Check sheet for the modelled part. Datum: model origin and axes. Units: mm. Give positions to 0.01 mm unless a question says otherwise; leave off trailing zeros. Order: outer loops, then holes, each group sorted by start corner. A loop starts at its lowest first (then second) coordinate and runs counter-clockwise, first axis right, second up. Notation, with made-up numbers: (-36, 8.25) -> (19, 8.25) arc R21 cw to (19, 22.25) -> close; hole circle Ø5 at (42.25, 45). An arc over 180 degrees is marked (long way). One line per question, with ' | ' between items.
```python
from build123d import *

# Parameters (mm, degrees)
SKETCH_1_R            = 1
SKETCH_1_R_2          = 11.2
SKETCH_1_R_3          = 4.05
SKETCH_1_R_4          = 3.5
SKETCH_1_R_5          = 8.2
SKETCH_1_R_6          = 4.2
EXTRUDE_1_DEPTH       = 7
SKETCH_6_R            = 21.8
SKETCH_6_R_2          = 8
CUT_EXTRUDE_3_DEPTH   = 4
SKETCH_7_R            = 3
CUT_EXTRUDE_4_DEPTH   = 6
SKETCH_13_R           = 1.75
CUT_EXTRUDE_4_2_DEPTH = 5


with BuildPart() as part:
    # Эскиз1 → Бобышка-Вытянуть1 (new body)
    with BuildSketch(Plane.XY):
        with BuildLine():
            Line((10, 0), (435, 0))
            ThreePointArc((435, 0), (442.071067812, 2.928932188), (445, 10))
            Line((445, 10), (445, 122.5))
            ThreePointArc((445, 122.5), (442.071067812, 129.571067812), (435, 132.5))
            Line((435, 132.5), (10, 132.5))
            ThreePointArc((10, 132.5), (2.928932188, 129.571067812), (0, 122.5))
            Line((0, 122.5), (0, 10))
            ThreePointArc((0, 10), (2.928932188, 2.928932188), (10, 0))
        make_face()
        with Locations((222.3, 105)):
            Circle(SKETCH_1_R, mode=Mode.SUBTRACT)
        with Locations((222.3, 66)):
            Circle(SKETCH_1_R_2, mode=Mode.SUBTRACT)
        with Locations((80, 66)):
            Circle(SKETCH_1_R_3, mode=Mode.SUBTRACT)
        with Locations((264, 66)):
            Circle(SKETCH_1_R_4, mode=Mode.SUBTRACT)
        with Locations((294, 66)):
            Circle(SKETCH_1_R_4, mode=Mode.SUBTRACT)
        with Locations((180.6, 66)):
            Circle(SKETCH_1_R_5, mode=Mode.SUBTRACT)
        with Locations((365, 66)):
            Circle(SKETCH_1_R_6, mode=Mode.SUBTRACT)
        with Locations((15.6, 66)):
            Circle(SKETCH_1_R_5, mode=Mode.SUBTRACT)
        with Locations((150.6, 66)):
            Circle(SKETCH_1_R_5, mode=Mode.SUBTRACT)
    extrude(amount=EXTRUDE_1_DEPTH)

    # Эскиз6 → Вырез-Вытянуть3 (cut)
    with BuildSketch(Plane.XY.offset(7)):
        with Locations((80, 66)):
            Circle(SKETCH_6_R)
        with Locations((365, 66)):
            Circle(SKETCH_6_R)
        with Locations((264, 66)):
            Circle(SKETCH_6_R_2)
        with Locations((294, 66)):
            Circle(SKETCH_6_R_2)
    extrude(amount=-CUT_EXTRUDE_3_DEPTH, mode=Mode.SUBTRACT)

    # Эскиз7 → Cut-Extrude 4 (cut)
    with BuildSketch(Plane(origin=(0, 0, 0), x_dir=(-1, 0, 0), z_dir=(0, 0, -1))):
        with Locations((-222.3, 105)):
            Circle(SKETCH_7_R)
    extrude(amount=-CUT_EXTRUDE_4_DEPTH, mode=Mode.SUBTRACT)

    # Эскиз13 → Cut-Extrude 4 2 (cut)
    with BuildSketch(Plane(origin=(0, 0, 0), x_dir=(-1, 0, 0), z_dir=(0, 0, -1))):
        with Locations((-17, 118.4)):
            Circle(SKETCH_13_R)
        with Locations((-17, 14.1)):
            Circle(SKETCH_13_R)
        with Locations((-428, 14.1)):
            Circle(SKETCH_13_R)
        with Locations((-428, 118.4)):
            Circle(SKETCH_13_R)
    extrude(amount=-CUT_EXTRUDE_4_2_DEPTH, mode=Mode.SUBTRACT)


solid = part.part
```
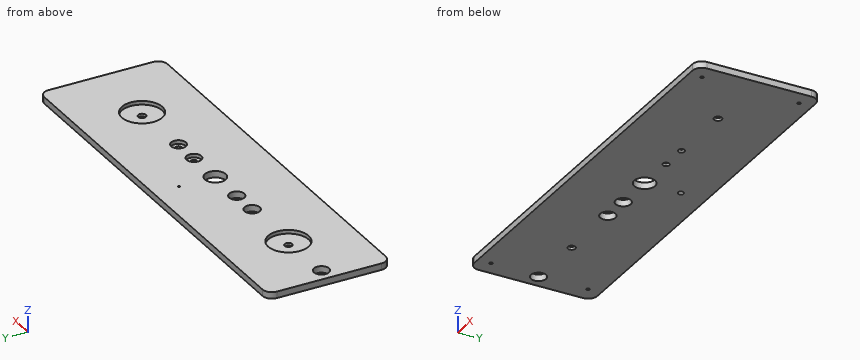
Q1. Section check D-D (x = 94). Enter the section's corners in (y, z), and give its area (3 significant figures).
Result sheet:
outline: (0, 0) -> (132.5, 0) -> (132.5, 7) -> (82.71, 7) -> (82.71, 3) -> (49.29, 3) -> (49.29, 7) -> (0, 7) -> close | area: 794 mm2
Q2. Section check A-A (x = 180.6). Enter the section's corners in (y, z).
Result sheet:
outline: (0, 0) -> (57.8, 0) -> (57.8, 7) -> (0, 7) -> close; (74.2, 0) -> (132.5, 0) -> (132.5, 7) -> (74.2, 7) -> close
Q3. Section check B-B (z = 1.5). Count the separate pieces of the cut face and the enclosed holes in it, and give its area (3 significant figures).
Result sheet:
separate pieces: 1 | enclosed holes: 13 | area: 57,600 mm2
Q4. Section check C-C (x = 379.5). Enter the section's corners in (y, z).
Result sheet:
outline: (0, 0) -> (132.5, 0) -> (132.5, 7) -> (82.28, 7) -> (82.28, 3) -> (49.72, 3) -> (49.72, 7) -> (0, 7) -> close
Q5. Thickness scan on line 1 (Y direction, x = 428, z = 2.35); line 2 (Y direction, x = 80, z = 2.05); line 3 (X direction, y = 85, z = 5). Record the ranges inside material, lowest first.
Result sheet:
line 1: y = 0 to 12.35, 15.85 to 116.65, 120.15 to 132.5 | line 2: y = 0 to 61.95, 70.05 to 132.5 | line 3: x = 0 to 69.31, 90.69 to 354.31, 375.69 to 445
Q6. Depth check by flat-ended pin: pin 1 Ø13 at (x, y) = (361.5, 66) entering from +Z. Enter the tip coordinate at first touch or a pass-through.
Result sheet:
pin 1: stops at z = 3
